from build123d import *

# Parameters (mm, degrees)
SKETCH1_R                      = 9.525
BOSS_EXTRUDE1_DEPTH            = 35
CHAMFER2_SIZE                  = 0.5
SKETCH2_W                      = 1
SKETCH2_H                      = 0.55
FILLET2_R                      = 0.25
M5X0_8_TAPPED_HOLE1_AT_2_COUNT = 2
M5X0_8_TAPPED_HOLE1_AT_2_PITCH = 21
M5X0_8_TAPPED_HOLE1_AT_3_COUNT = 2
M5X0_8_TAPPED_HOLE1_AT_3_PITCH = 35
M5X0_8_TAPPED_HOLE1_AT_4_COUNT = 2
M5X0_8_TAPPED_HOLE1_AT_4_PITCH = 28
CHAMFER3_SIZE                  = 0.5


with BuildPart() as part:
    # Sketch1 → Boss-Extrude1 (new body)
    with BuildSketch(Plane.XY):
        with BuildLine():
            Line((18.646446609, -1.146446609), (19.853553391, -2.353553391))
            ThreePointArc((19.853553391, -2.353553391), (19.961939766, -2.515765065), (20, -2.707106781))
            Line((20, -2.707106781), (20, -12.5))
            Line((20, -12.5), (19.5, -13))
            Line((19.5, -13), (7.707106781, -13))
            ThreePointArc((7.707106781, -13), (7.515765065, -12.961939766), (7.353553391, -12.853553391))
            Line((7.353553391, -12.853553391), (7.292893219, -12.792893219))
            ThreePointArc((7.292893219, -12.792893219), (6.96846987, -12.576120467), (6.585786438, -12.5))
            Line((6.585786438, -12.5), (-6.585786438, -12.5))
            ThreePointArc((-6.585786438, -12.5), (-6.96846987, -12.576120467), (-7.292893219, -12.792893219))
            Line((-7.292893219, -12.792893219), (-7.353553391, -12.853553391))
            ThreePointArc((-7.353553391, -12.853553391), (-7.515765065, -12.961939766), (-7.707106781, -13))
            Line((-7.707106781, -13), (-19.5, -13))
            Line((-19.5, -13), (-20, -12.5))
            Line((-20, -12.5), (-20, -2.707106781))
            ThreePointArc((-20, -2.707106781), (-19.961939766, -2.515765065), (-19.853553391, -2.353553391))
            Line((-19.853553391, -2.353553391), (-18.646446609, -1.146446609))
            ThreePointArc((-18.646446609, -1.146446609), (-18.538060234, -0.984234935), (-18.5, -0.792893219))
            Line((-18.5, -0.792893219), (-18.5, 7.5))
            ThreePointArc((-18.5, 7.5), (-18.353553391, 7.853553391), (-18, 8))
            Line((-18, 8), (-10.707106781, 8))
            ThreePointArc((-10.707106781, 8), (-10.515765065, 8.038060234), (-10.353553391, 8.146446609))
            Line((-10.353553391, 8.146446609), (-5.792893219, 12.707106781))
            ThreePointArc((-5.792893219, 12.707106781), (-5.46846987, 12.923879533), (-5.085786438, 13))
            Line((-5.085786438, 13), (5.085786438, 13))
            ThreePointArc((5.085786438, 13), (5.46846987, 12.923879533), (5.792893219, 12.707106781))
            Line((5.792893219, 12.707106781), (10.353553391, 8.146446609))
            ThreePointArc((10.353553391, 8.146446609), (10.515765065, 8.038060234), (10.707106781, 8))
            Line((10.707106781, 8), (18, 8))
            ThreePointArc((18, 8), (18.353553391, 7.853553391), (18.5, 7.5))
            Line((18.5, 7.5), (18.5, -0.792893219))
            ThreePointArc((18.5, -0.792893219), (18.538060234, -0.984234935), (18.646446609, -1.146446609))
        make_face()
        with Locations(Location((0, 0, 0), (0, 0, 180))):
            Circle(SKETCH1_R, mode=Mode.SUBTRACT)
    extrude(amount=BOSS_EXTRUDE1_DEPTH)

    # Chamfer2
    chamfer2_edges = [part.edges().sort_by_distance(p)[0] for p in [
        (9.525, 0, 0),
        (9.525, 0, 35),
    ]]
    chamfer(chamfer2_edges, length=CHAMFER2_SIZE)

    # Sketch2 → Cut-Revolve1 (revolve, cut)
    with BuildSketch(Plane(origin=(0, 0, 0), x_dir=(0, 0, -1), z_dir=(1, 0, 0)), mode=Mode.PRIVATE) as cut_revolve1_sk:
        with Locations((-32.5, -9.775)):
            Rectangle(SKETCH2_W, SKETCH2_H)
        with Locations((-2.5, -9.775)):
            Rectangle(SKETCH2_W, SKETCH2_H)
    revolve(cut_revolve1_sk.sketch.rotate(Axis((0, 0, 0), (0, 0, 1)), 270), axis=Axis((0, 0, 0), (0, 0, 1)), mode=Mode.SUBTRACT)

    # Fillet2
    fillet2_edges = [part.edges().sort_by_distance(p)[0] for p in [
        (9.525, 0, 33),
        (9.525, 0, 32),
        (9.525, 0, 3),
        (9.525, 0, 2),
    ]]
    fillet(fillet2_edges, radius=FILLET2_R)

    # Sketch5 → M5x0.8 Tapped Hole1 (revolve, cut)
    with BuildSketch(Plane(origin=(-14, -13, 28), x_dir=(0, 0, -1), z_dir=(1, 0, 0))):
        Polygon((0, 0), (0, 21), (3, 21), (2.15, 20.15), (2.15, 1.35), (3.5, 0), align=None)
    m5x0_8_tapped_hole1 = revolve(axis=Axis((-14, -19.35, 28), (0, 1, 0)), mode=Mode.SUBTRACT)

    # M5x0.8 Tapped Hole1 at 2: M5x0.8 Tapped Hole1 ×2
    with Locations(*[(0, 0, -i * M5X0_8_TAPPED_HOLE1_AT_2_PITCH) for i in range(1, M5X0_8_TAPPED_HOLE1_AT_2_COUNT)]):
        add(m5x0_8_tapped_hole1, mode=Mode.SUBTRACT)

    # M5x0.8 Tapped Hole1 at 3: M5x0.8 Tapped Hole1 ×2
    with Locations(*[Vector(0.8, 0, -0.6) * (i * M5X0_8_TAPPED_HOLE1_AT_3_PITCH) for i in range(1, M5X0_8_TAPPED_HOLE1_AT_3_COUNT)]):
        add(m5x0_8_tapped_hole1, mode=Mode.SUBTRACT)

    # M5x0.8 Tapped Hole1 at 4: M5x0.8 Tapped Hole1 ×2
    with Locations(*[(i * M5X0_8_TAPPED_HOLE1_AT_4_PITCH, 0, 0) for i in range(1, M5X0_8_TAPPED_HOLE1_AT_4_COUNT)]):
        add(m5x0_8_tapped_hole1, mode=Mode.SUBTRACT)

    # Chamfer3
    chamfer3_edges = [part.edges().sort_by_distance(p)[0] for p in [
        (18.353553391, 7.853553391, 0),
        (18.5, 3.353553391, 0),
        (18.538060234, -0.984234935, 0),
        (19.25, -1.75, 0),
        (19.961939766, -2.515765065, 0),
        (20, -7.603553391, 0),
        (-20, -7.603553391, 0),
        (-19.961939766, -2.515765065, 0),
        (-19.25, -1.75, 0),
        (-18.538060234, -0.984234935, 0),
        (-18.5, 3.353553391, 0),
        (-18.353553391, 7.853553391, 0),
        (-14.353553391, 8, 0),
        (-10.515765065, 8.038060234, 0),
        (-8.073223305, 10.426776695, 0),
        (-5.46846987, 12.923879533, 0),
        (0, 13, 0),
        (5.46846987, 12.923879533, 0),
        (8.073223305, 10.426776695, 0),
        (10.515765065, 8.038060234, 0),
        (14.353553391, 8, 0),
    ]]
    chamfer(chamfer3_edges, length=CHAMFER3_SIZE - 0.0001)  # a hair under: the kernel refuses the full size
    chamfer3_2_edges = [part.edges().sort_by_distance(p)[0] for p in [
        (13.603553391, -13, 0),
        (7.515765065, -12.961939766, 0),
        (7.323223305, -12.823223305, 0),
        (6.96846987, -12.576120467, 0),
        (0, -12.5, 0),
        (-6.96846987, -12.576120467, 0),
        (-7.323223305, -12.823223305, 0),
        (-7.515765065, -12.961939766, 0),
        (-13.603553391, -13, 0),
    ]]
    chamfer(chamfer3_2_edges, length=CHAMFER3_SIZE - 0.0001)  # a hair under: the kernel refuses the full size
    chamfer3_3_edges = [part.edges().sort_by_distance(p)[0] for p in [
        (18.353553391, 7.853553391, 35),
        (18.5, 3.353553391, 35),
        (18.538060234, -0.984234935, 35),
        (19.25, -1.75, 35),
        (19.961939766, -2.515765065, 35),
        (20, -7.603553391, 35),
        (-20, -7.603553391, 35),
        (-19.961939766, -2.515765065, 35),
        (-19.25, -1.75, 35),
        (-18.538060234, -0.984234935, 35),
        (-18.5, 3.353553391, 35),
        (-18.353553391, 7.853553391, 35),
        (-14.353553391, 8, 35),
        (-10.515765065, 8.038060234, 35),
        (-8.073223305, 10.426776695, 35),
        (-5.46846987, 12.923879533, 35),
        (0, 13, 35),
        (5.46846987, 12.923879533, 35),
        (8.073223305, 10.426776695, 35),
        (10.515765065, 8.038060234, 35),
        (14.353553391, 8, 35),
    ]]
    chamfer(chamfer3_3_edges, length=CHAMFER3_SIZE - 0.0001)  # a hair under: the kernel refuses the full size
    chamfer3_4_edges = [part.edges().sort_by_distance(p)[0] for p in [
        (13.603553391, -13, 35),
        (7.515765065, -12.961939766, 35),
        (7.323223305, -12.823223305, 35),
        (6.96846987, -12.576120467, 35),
        (0, -12.5, 35),
        (-6.96846987, -12.576120467, 35),
        (-7.323223305, -12.823223305, 35),
        (-7.515765065, -12.961939766, 35),
        (-13.603553391, -13, 35),
    ]]
    chamfer(chamfer3_4_edges, length=CHAMFER3_SIZE - 0.0001)  # a hair under: the kernel refuses the full size


solid = part.part
Verification items for the finished model (mm, model axes). Coordinates: 2 decimals unless noted, no trailing zeros. Order: outer loops, then holes, each group sorted by start corner. A loop starts at its lowest first (then second) coordinate and runs counter-clockwise, first axis right, second up.
1. Scan lines: line 1 (Z direction, x = 14, y = -11); line 2 (Y direction, x = 0, z = 33.7) (3 decimals); line 3 (Z direction, x = -4, y = -9). Record each from-to range of solid material in increasing order.
Results found:
line 1: z = 0 to 4.85, 9.15 to 25.85, 30.15 to 35
line 2: y = -12.5 to -9.525, 9.525 to 13
line 3: z = 0.18 to 2, 3 to 32, 33 to 34.82
2. Go/stop test with flat-tipped pins: pin 1 Ø8 at (x, z) = (-1.5, 20.5) entering from -Y; pin 2 Ø2 at (y, z) = (6.5, 29) entering from -X; pin 3 Ø5.5 at (x, z) = (-14, 7) entering from -Y. Record where each tip stops, or that it passes through.
Results found:
pin 1: stops at y = -12.5
pin 2: stops at x = -18.5
pin 3: stops at y = -12.25
3. Sectioned sample at B-B, the plane x = 14. Record the cut outline in (y, z).
Results found:
outline: (-13, 0.5) - (-12.5, 0) - (7.5, 0) - (8, 0.5) - (8, 4) - (7.15, 4.85) - (-11.65, 4.85) - (-13, 3.5) - close; (-13, 10.5) - (-11.65, 9.15) - (7.15, 9.15) - (8, 10) - (8, 25) - (7.15, 25.85) - (-11.65, 25.85) - (-13, 24.5) - close; (-13, 31.5) - (-11.65, 30.15) - (7.15, 30.15) - (8, 31) - (8, 34.5) - (7.5, 35) - (-12.5, 35) - (-13, 34.5) - close
4. Sectioned sample at C-C, the plane z = 7. Give the number of separate pieces and of enclosed holes in the cut face, and give its area (3 significant figures).
Results found:
separate pieces: 3
enclosed holes: 1
area: 412 mm2
5. Release check for a two-part mould opening along Z. For faces 1 (the face through (0, -11, 35)), 2 (the face through (15.91, -2.38, 6.01)), 3 (the face through (0, 13, 17)) record: +Z half, -Z half, draft (parallel to the pull), parting line (faces both ways), or undercut.
Results found:
face 1: +Z half
face 2: undercut
face 3: draft
